from build123d import *

# Parameters (mm, degrees)
SKETCH1_R           = 2.5
BOSS_EXTRUDE1_DEPTH = 10
SKETCH3_R           = 10
SKETCH3_R_2         = 2.5
BOSS_EXTRUDE2_DEPTH = 4
SKETCH4_R           = 10
SKETCH4_R_2         = 2.5
BOSS_EXTRUDE3_DEPTH = 2
SKETCH4_2_R         = 10
SKETCH4_2_R_2       = 2.5
CUT_EXTRUDE1_DEPTH  = 4


with BuildPart() as part:
    # Sketch1 → Boss-Extrude1 (new body)
    with BuildSketch(Plane(origin=(0, 0, 0), x_dir=(1, 0, 0), z_dir=(0, 1, 0))):
        Circle(SKETCH1_R)
        with BuildLine():
            Line((-1.242447099, 0.840431559), (0.968768208, 1.14513458))
            ThreePointArc((0.968768208, 1.14513458), (0.204756352, -1.485907091), (-1.242447099, 0.840431559))
        make_face(mode=Mode.SUBTRACT)
    extrude(amount=BOSS_EXTRUDE1_DEPTH)

    # Sketch3 → Boss-Extrude2 (add)
    with BuildSketch(Plane(origin=(0, 10, 0), x_dir=(1, 0, 0), z_dir=(0, 1, 0))):
        Circle(SKETCH3_R)
        Circle(SKETCH3_R_2, mode=Mode.SUBTRACT)
    extrude(amount=-BOSS_EXTRUDE2_DEPTH)

    # Sketch4 → Boss-Extrude3 (add)
    with BuildSketch(Plane.XZ.offset(-6)):
        Circle(SKETCH4_R)
        Circle(SKETCH4_R_2, mode=Mode.SUBTRACT)
    extrude(amount=BOSS_EXTRUDE3_DEPTH)

    # Sketch4<2> → Cut-Extrude1 (cut)
    with BuildSketch(Plane.XZ.offset(-6)):
        Circle(SKETCH4_2_R)
        Circle(SKETCH4_2_R_2, mode=Mode.SUBTRACT)
    extrude(amount=-CUT_EXTRUDE1_DEPTH, mode=Mode.SUBTRACT)


solid = part.part
Input: part model. Units: mm. Frame: model coordinates. A direction names the side the tool comes from. Coordinates: 2 decimals unless noted, no trailing zeros. Loops run counter-clockwise (first coordinate to the right, second up) from the corner with the lowest first, then second, coordinate; pieces in that order, holes last. Notation, with made-up numbers: (5.5, -16.5) -> (21.5, -16.5) arc R14 ccw to (21.5, 9.5) -> close; hole circle Ø2 at (84, 26.25). An arc over 180 degrees is marked (long way). One line per item, written item: value.
(1) Draft query along X for faces 1 (the face through (-2.17, 5.01, -9.76)), 2 (the face through (-0.15, 4.93, -0.99)), 3 (the face through (0.25, 4.93, 1.48)), 4 (the face through (2, 4, -2)). Return one class per face: pulls with the +X half, pulls with the -X half, needs draft (parallel to the pull), parting line crosses it, or undercut.
Answer below:
face 1: parting line crosses it
face 2: undercut
face 3: undercut
face 4: needs draft
(2) Pin query (flat end, axial travel): pin 1 Ø2 at (x, y) = (-6, 4.5) entering from -Z; pin 2 Ø6 at (y, z) = (5, -6) entering from -X; pin 3 Ø8 at (x, z) = (-7, -5) entering from +Y. Return the tip coordinate at first contact, or that it passes through.
Answer below:
pin 1: stops at z = -8.66
pin 2: stops at x = -9.54
pin 3: stops at y = 6
(3) Cut plane B-B (x = 0). Output: boundary loops of the cut face in (y, z), then the cut area to 3 significant figures.
Answer below:
outline: (0, -2.5) -> (4, -2.5) -> (4, -10) -> (6, -10) -> (6, -2.5) -> (10, -2.5) -> (10, -1.01) -> (0, -1.01) -> close; (0, 1.5) -> (10, 1.5) -> (10, 2.5) -> (6, 2.5) -> (6, 10) -> (4, 10) -> (4, 2.5) -> (0, 2.5) -> close
area: 54.9 mm2
(4) Set-up query: faces 5 (the face through (-0.6, 10, -1.1)), 6 (the face through (2, 6, -2)), 7 (the face through (-0.54, 1.97, 2.44)). Return all of +Z, -Z, +X, -X, +Y, -Y with unobstructed straight access to the full face (end or side cutting, diameter ignored); none if empty.
Answer below:
face 5: +Z, -Z, +X, -X, +Y
face 6: +Y
face 7: -Y
(5) Cut plane A-A (z = 0). Output: boundary loops of the cut face in (x, y).
Answer below:
outline: (-10, 4) -> (-2.5, 4) -> (-2.5, 0) -> (-1.5, 0) -> (-1.5, 10) -> (-2.5, 10) -> (-2.5, 6) -> (-10, 6) -> close; (1.5, 0) -> (2.5, 0) -> (2.5, 4) -> (10, 4) -> (10, 6) -> (2.5, 6) -> (2.5, 10) -> (1.5, 10) -> close
(6) Ray query, line 1 along Y through (x, z) = (-3.75, -6.5); line 2 along X through (y, z) = (8.5, 2); line 3 along X through (y, z) = (5.25, 3.25). Return the intervals inside material, ascending.
Answer below:
line 1: y = 4 to 6
line 2: x = -1.5 to 1.5
line 3: x = -9.46 to 9.46
(7) Cut plane D-D (x = -5). Output: boundary loops of the cut face in (y, z), then the cut area to 3 significant figures.
Answer below:
outline: (4, -8.66) -> (6, -8.66) -> (6, 8.66) -> (4, 8.66) -> close
area: 34.6 mm2
(8) Cut plane C-C (y = 7). Output: boundary loops of the cut face in (x, z), then the cut area to 3 significant figures.
Answer below:
outline: circle Ø5 at (0, 0); hole (-1.24, -0.84) -> (0.97, -1.15) arc R1.5 ccw (long way) to start
area: 13.3 mm2
